from build123d import *

# Parameters (mm, degrees)
SKETCH1_W           = 12
SKETCH1_H           = 12
SKETCH1_W_2         = 9
SKETCH1_H_2         = 9
BOSS_EXTRUDE1_DEPTH = 48
SKETCH3_W           = 20
SKETCH3_H           = 20
BOSS_EXTRUDE2_DEPTH = 2
SKETCH4_W           = 20
SKETCH4_H           = 20
BOSS_EXTRUDE3_DEPTH = 2


with BuildPart() as part:
    # Sketch1 → Boss-Extrude1 (new body)
    with BuildSketch(Plane(origin=(0, 0, 0), x_dir=(1, 0, 0), z_dir=(0, 1, 0))):
        Rectangle(SKETCH1_W, SKETCH1_H)
        Rectangle(SKETCH1_W_2, SKETCH1_H_2, mode=Mode.SUBTRACT)
    extrude(amount=BOSS_EXTRUDE1_DEPTH)

    # Sketch3 → Boss-Extrude2 (add)
    with BuildSketch(Plane(origin=(0, 0, 0), x_dir=(1, 0, 0), z_dir=(0, 1, 0))):
        Rectangle(SKETCH3_W, SKETCH3_H)
    extrude(amount=-BOSS_EXTRUDE2_DEPTH)

    # Sketch4 → Boss-Extrude3 (add)
    with BuildSketch(Plane(origin=(0, 48, 0), x_dir=(1, 0, 0), z_dir=(0, 1, 0))):
        Rectangle(SKETCH4_W, SKETCH4_H)
    extrude(amount=BOSS_EXTRUDE3_DEPTH)


solid = part.part
The listing builds one solid part. Answer for the finished solid, in the listing's coordinates (mm). A direction names the side the tool comes from. Give positions to 0.01 mm unless a question says otherwise; leave off trailing zeros. Loops run counter-clockwise (first coordinate to the right, second up) from the corner with the lowest first, then second, coordinate; pieces in that order, holes last.
Item 1: A cutting plane is placed at B-B (z = 8). Give the vertices of the cut face in (x, y), then the cut area to 3 significant figures.
Derived:
outline: (-10, -2) - (10, -2) - (10, 0) - (-10, 0) - close; (-10, 48) - (10, 48) - (10, 50) - (-10, 50) - close
area: 80.0 mm2
Item 2: Each of these flat-tipped pins is pushed along its axis until it touches: pin 1 Ø2 at (x, y) = (3.5, 18) entering from +Z; pin 2 Ø4.5 at (y, z) = (13.5, -1) entering from -X; pin 3 Ø5 at (y, z) = (44, 1) entering from +X. Where does it stop, or does it pass through?
Derived:
pin 1: stops at z = 6
pin 2: stops at x = -6
pin 3: stops at x = 6
Item 3: A cutting plane is placed at D-D (x = 2.5). Give the vertices of the cut face in (y, z).
Derived:
outline: (-2, -10) - (0, -10) - (0, -6) - (48, -6) - (48, -10) - (50, -10) - (50, 10) - (48, 10) - (48, 6) - (0, 6) - (0, 10) - (-2, 10) - close; hole (0, -4.5) - (48, -4.5) - (48, 4.5) - (0, 4.5) - close
Item 4: Determine the mould class of faces 1 (the flat face through (0, -2, 0)), 2 (the flat face through (6, 24, 0)), 3 (the flat face through (10, -1, 0)) for opening direction Y: +Y half, -Y half, draft (parallel to the pull), parting line (faces both ways), or undercut.
Derived:
face 1: -Y half
face 2: undercut
face 3: draft
Item 5: A tool of negligible diameter and unlimited length cuts with its end or side. For faces 4 (the flat face through (0, 50, 0)), 5 (the flat face through (-4.5, 24, 0)), 6 (the flat face through (0, 24, 6)), 7 (the flat face through (0, 49, -10)), 8 (the flat face through (0, 24, -6)), from which of +Z, -Z, +X, -X, +Y, -Y can it reach the whole face along a straight path? Write none if from no direction.
Derived:
face 4: +Z, -Z, +X, -X, +Y
face 5: none
face 6: +Z, +X, -X
face 7: -Z, +X, -X, +Y, -Y
face 8: -Z, +X, -X
Item 6: A cutting plane is placed at A-A (x = -7.5). Give the vertices of the cut face in (y, z).
Derived:
outline: (-2, -10) - (0, -10) - (0, 10) - (-2, 10) - close; (48, -10) - (50, -10) - (50, 10) - (48, 10) - close
Item 7: A cutting plane is placed at C-C (y = 31.5). Give the vertices of the cut face in (x, z), then the cut area to 3 significant figures.
Derived:
outline: (-6, -6) - (6, -6) - (6, 6) - (-6, 6) - close; hole (-4.5, -4.5) - (4.5, -4.5) - (4.5, 4.5) - (-4.5, 4.5) - close
area: 63.0 mm2
Item 8: Find the intervals of material crossed by line 1 along Z through (x, y) = (0.5, 12.5); line 2 along Y through (x, z) = (3, -3.5), in increasing order.
Derived:
line 1: z = -6 to -4.5, 4.5 to 6
line 2: y = -2 to 0, 48 to 50
